Design review of the part built by this model. Coordinates are the model's own, in mm. A direction names the side the tool comes from. Coordinates: 2 decimals unless noted, no trailing zeros. Write each loop counter-clockwise with the first axis right and the second up, starting at its lowest first coordinate (ties: lowest second). Pieces come first, ordered by that corner, then holes.
Q1. For probe 1 along Y at (x, z) = (-17.75, -4.45) (3 decimals); probe 2 along Y at (x, z) = (17.75, -2.6); probe 3 along Z at (x, y) = (13.5, 1), list the stretches that pass through material, from the lowest coordinate up.
Q2. Take a section at C-C (z = 6). Give the boundary of the cut face in (x, y), and give its area (3 significant figures).
Q3. Take a section at A-A (x = 0). Give the boundary of the cut face in (y, z).
Q4. Take a section at B-B (x = 15.5). Give the boundary of the cut face in (y, z).
Q5. Machinability: for faces 1 (the flat face through (13, -9.3, -4)), 2 (the flat face through (-13, -9.3, -4)), 3 (the flat face through (5, 0, 11.5)), which of the approach directions +Z, -Z, +X, -X, +Y, -Y give a long, thin tool a straight path to every point of the face, cutting with its end or side? Answer none if there is none.
Q6. Mouldability with a two-part tool opening along X and no side actions: class faces 4 (the cylindrical face through (-22.445, 0.207, -1.775)), 5 (the cylindrical face through (-1.658, -7.468, 10.341)), 6 (the flat face through (0, 0, -7.8)) as pulls with the +X half, pulls with the -X half, needs draft (parallel to the pull), parting line crosses it, or undercut.
Q7. Insertion check: pin 1 (7.5 mm diameter, centred on x = 17.75, y = 0, fed in from +Z); pin 2 (12 mm diameter, centred on x = 8, y = -8, fed in from +Z); pin 3 (1 mm diameter, centred on y = -5.5, z = 30.5, fed in from +X); pin 4 (4 mm diameter, centred on x = 12, z = -4.5, fed in from -Y). Each pin has a flat end and moves straight along its axis. Give the tip position at first contact, or say it passes through.
Q8. Take a section at D-D (z = 27). Give the boundary of the cut face in (x, y), and give its area (3 significant figures).
```python
from build123d import *
from build123d import SkipClean  # not in build123d's __all__

# Parameters (mm, degrees)
F0_R           = 7.65
F0_R_2         = 4.65
F1_DEPTH       = 7.8
F2_DEPTH       = 9.7
F3_DEPTH       = 11.5
F4_DEPTH       = 35
F5_D           = 5.75
F5_CBORE_D     = 9.4
F5_CBORE_DEPTH = 3.6
F6_R           = 0.5
F7_R           = 1.5


# Not quite as in the source:
# - after a boolean that leaves OpenCascade's solid faulty, fix() repairs it


with BuildPart() as f1:
    # F0 (on Top) → F1 (new body)
    with BuildSketch(Plane.XY):
        with BuildLine():
            ThreePointArc((-8.3522452071, -9.3), (-12.5, 0), (-8.3522452071, 9.3))
            Line((-8.3522452071, 9.3), (-17.45, 9.3))
            ThreePointArc((-17.45, 9.3), (-24.026093065, 6.576093065), (-26.75, 0))
            ThreePointArc((-26.75, 0), (-24.026093065, -6.576093065), (-17.45, -9.3))
            Line((-17.45, -9.3), (-8.3522452071, -9.3))
        make_face()
        with BuildLine():
            ThreePointArc((12.5, 0), (11.4160646698, 5.0915093494), (8.3522452071, 9.3))
            Line((8.3522452071, 9.3), (-8.3522452071, 9.3))
            ThreePointArc((-8.3522452071, 9.3), (-12.5, 0), (-8.3522452071, -9.3))
            Line((-8.3522452071, -9.3), (8.3522452071, -9.3))
            ThreePointArc((8.3522452071, -9.3), (11.4160646698, -5.0915093494), (12.5, 0))
        make_face()
        Circle(F0_R, mode=Mode.SUBTRACT)
        Circle(F0_R)
        Circle(F0_R_2, mode=Mode.SUBTRACT)
        Circle(F0_R_2)
        with BuildLine():
            ThreePointArc((26.75, 0), (24.026093065, 6.576093065), (17.45, 9.3))
            Line((17.45, 9.3), (8.3522452071, 9.3))
            ThreePointArc((8.3522452071, 9.3), (11.4160646698, 5.0915093494), (12.5, 0))
            ThreePointArc((12.5, 0), (11.4160646698, -5.0915093494), (8.3522452071, -9.3))
            Line((8.3522452071, -9.3), (17.45, -9.3))
            ThreePointArc((17.45, -9.3), (24.026093065, -6.576093065), (26.75, 0))
        make_face()
        with BuildLine():
            Line((-8.3522452071, 9.3), (8.3522452071, 9.3))
            ThreePointArc((8.3522452071, 9.3), (0, 12.5), (-8.3522452071, 9.3))
        make_face()
        with BuildLine():
            ThreePointArc((-8.3522452071, -9.3), (0, -12.5), (8.3522452071, -9.3))
            Line((8.3522452071, -9.3), (-8.3522452071, -9.3))
        make_face()
    extrude(amount=-F1_DEPTH)

    # F0 (on Top) → F2 (join)
    with BuildSketch(Plane.XY):
        with BuildLine():
            Line((-8.3522452071, 9.3), (8.3522452071, 9.3))
            ThreePointArc((8.3522452071, 9.3), (0, 12.5), (-8.3522452071, 9.3))
        make_face()
        with BuildLine():
            ThreePointArc((-8.3522452071, -9.3), (0, -12.5), (8.3522452071, -9.3))
            Line((8.3522452071, -9.3), (-8.3522452071, -9.3))
        make_face()
        with BuildLine():
            ThreePointArc((12.5, 0), (11.4160646698, 5.0915093494), (8.3522452071, 9.3))
            Line((8.3522452071, 9.3), (-8.3522452071, 9.3))
            ThreePointArc((-8.3522452071, 9.3), (-12.5, 0), (-8.3522452071, -9.3))
            Line((-8.3522452071, -9.3), (8.3522452071, -9.3))
            ThreePointArc((8.3522452071, -9.3), (11.4160646698, -5.0915093494), (12.5, 0))
        make_face()
        Circle(F0_R, mode=Mode.SUBTRACT)
        Circle(F0_R)
        Circle(F0_R_2, mode=Mode.SUBTRACT)
        Circle(F0_R_2)
    with SkipClean():  # cleaning this boolean's faces spoils the solid; the shape is the same uncleaned
        extrude(amount=F2_DEPTH)

    # F0 (on Top) → F3 (join)
    with BuildSketch(Plane.XY):
        Circle(F0_R)
        Circle(F0_R_2, mode=Mode.SUBTRACT)
        Circle(F0_R_2)
    extrude(amount=F3_DEPTH)

    add(f1.part.fix(), mode=Mode.REPLACE)

    # F0 (on Top) → F4 (join)
    with BuildSketch(Plane.XY):
        Circle(F0_R_2)
    extrude(amount=F4_DEPTH)

    # F5 (through all)
    with Locations(Plane.XY):
        with Locations((-17.75, 0), (17.75, 0)):
            CounterBoreHole(F5_D / 2, F5_CBORE_D / 2, F5_CBORE_DEPTH)

    # F6
    f6_edges = [f1.edges().sort_by_distance(p)[0] for p in [
        (8.352245, -9.3, 9.7),
        (-7.65, 0, 11.5),
    ]]
    fillet(f6_edges, radius=F6_R)

    # F7
    f7_edges = [f1.edges().sort_by_distance(p)[0] for p in [
        (-4.65, 0, 35),
    ]]
    fillet(f7_edges, radius=F7_R)


solid = f1.part
```
Response:
1. probe 1: y = -9.295 to -2.875, 2.875 to 9.295
1. probe 2: y = -9.3 to -4.7, 4.7 to 9.3
1. probe 3: z = -7.8 to -3.6
2. outline: circle Ø25 at (0, 0)
2. area: 491 mm2
3. outline: (-12.5, -7.8) - (12.5, -7.8) - (12.5, 9.2) arc R0.5 ccw to (12, 9.7) - (7.65, 9.7) - (7.65, 11) arc R0.5 ccw to (7.15, 11.5) - (4.65, 11.5) - (4.65, 33.5) arc R1.5 ccw to (3.15, 35) - (-3.15, 35) arc R1.5 ccw to (-4.65, 33.5) - (-4.65, 11.5) - (-7.15, 11.5) arc R0.5 ccw to (-7.65, 11) - (-7.65, 9.7) - (-12, 9.7) arc R0.5 ccw to (-12.5, 9.2) - close
4. outline: (-9.3, -7.8) - (-1.79, -7.8) - (-1.79, -3.6) - (-4.13, -3.6) - (-4.13, 0) - (-9.3, 0) - close; (1.79, -7.8) - (9.3, -7.8) - (9.3, 0) - (4.13, 0) - (4.13, -3.6) - (1.79, -3.6) - close
5. face 1: +Z, -Z, +X, -Y
5. face 2: +Z, -Z, -X, -Y
5. face 3: +Z
6. face 4: undercut
6. face 5: parting line crosses it
6. face 6: needs draft
7. pin 1: stops at z = -3.6
7. pin 2: stops at z = 11.5
7. pin 3: passes through
7. pin 4: stops at y = -9.3
8. outline: circle Ø9.3 at (0, 0)
8. area: 67.9 mm2
